```python
from build123d import *

# Parameters (mm, degrees)
BOSS_EXTRUDE1_DEPTH = 2.54
BOSS_EXTRUDE2_DEPTH = 6.35


with BuildPart() as part:
    # Sketch1 → Revolve1 (revolve)
    with BuildSketch(Plane.XY):
        with BuildLine():
            Line((0, -13.880770422), (0, -18.033881925))
            Line((0, -18.033881925), (17.78, -18.033881925))
            Line((17.78, -18.033881925), (17.78, -8.528719197))
            Line((17.78, -8.528719197), (15.24, -8.528719197))
            Line((15.24, -8.528719197), (15.24, -15.493881925))
            Line((15.24, -15.493881925), (12.7, -15.493881925))
            ThreePointArc((12.7, -15.493881925), (6.401018058, -14.285661851), (0, -13.880770422))
        make_face()
    revolve(axis=Axis((0, -13.880770422, 0), (0, -1, 0)))

    # Sketch2 → Boss-Extrude1 (add)
    with BuildSketch(Plane.XZ.offset(18.033881925)):
        Polygon((28.413494599, 0), (8.780252701, 27.022839189), (-22.987, 16.701033091), (-22.987, -16.701033091), (8.780252701, -27.022839189), align=None)
    extrude(amount=-BOSS_EXTRUDE1_DEPTH)

    # Sketch3 → Boss-Extrude2 (add)
    with BuildSketch(Plane(origin=(0, -15.493881925, 0), x_dir=(1, 0, 0), z_dir=(0, 1, 0))):
        Polygon((28.413494599, 0), (8.780252701, 27.022839189), (-22.987, 16.701033091), (-22.987, -16.701033091), (8.780252701, -27.022839189), align=None)
        Polygon((25.273881936, 0), (7.810059032, 24.036890107), (-20.447, 14.85561507), (-20.447, -14.85561507), (7.810059032, -24.036890107), align=None, mode=Mode.SUBTRACT)
    extrude(amount=BOSS_EXTRUDE2_DEPTH)


solid = part.part
```
Read the model definition and answer for the solid it produces. Units are mm, in the model's axes. A direction names the side the tool comes from. Round coordinates to 2 decimals unless told otherwise and drop trailing zeros. Write each loop counter-clockwise with the first axis right and the second up, starting at its lowest first coordinate (ties: lowest second). Pieces come first, ordered by that corner, then holes. Notation, with made-up numbers: (22, 59.5) - (39, 59.5) arc R19 ccw to (39, 71.5) - close; hole circle Ø8 at (75.5, -35.5). An arc over 180 degrees is marked (long way). One line per item, written item: value.
Q1. Each of these flat-tipped pins is pushed along its axis until it touches: P1, Ø13.5, axis at x = 3.5, z = 5, coming from the +Y side; P2, Ø1.5, axis at x = 1, y = -13, coming from the +Z side; P3, Ø5, axis at y = -13, z = -7.5, coming from the +X side. Where does it stop, or does it pass through?
The answers:
P1: stops at y = -13.88
P2: stops at z = 24.74
P3: stops at x = 24.78
Q2. Find section C-C (z = -2). Determine the outline of the cut face in (x, y), and give its area (3 significant figures).
The answers:
outline: (-22.99, -18.03) - (26.96, -18.03) - (26.96, -9.14) - (23.82, -9.14) - (23.82, -15.49) - (17.67, -15.49) - (17.67, -8.53) - (15.11, -8.53) - (15.11, -15.49) - (12.54, -15.49) arc R50.76 ccw to (-12.54, -15.49) - (-15.11, -15.49) - (-15.11, -8.53) - (-17.67, -8.53) - (-17.67, -15.49) - (-20.45, -15.49) - (-20.45, -9.14) - (-22.99, -9.14) - close
area: 225 mm2
Q3. Which of the six approach directions +Z, -Z, +X, -X, +Y, -Y give full straight-line access (tool end or side, diameter ignored) to faces 1 (the flat face through (-8, -8.529, 13.3)), 2 (the cylindrical face through (-3.3, -12.06, -14.88))?
The answers:
face 1: +Z, -Z, +X, -X, +Y
face 2: +Y
Q4. Find section A-A (y = -10.5). Determine the outline of the cut face in (x, z), and give its area (3 significant figures).
The answers:
outline: (-22.99, -16.7) - (8.78, -27.02) - (28.41, 0) - (8.78, 27.02) - (-22.99, 16.7) - close; circle Ø35.56 at (0, 0); hole (-20.45, -14.86) - (7.81, -24.04) - (25.27, 0) - (7.81, 24.04) - (-20.45, 14.86) - close; hole circle Ø30.48 at (0, 0)
area: 664 mm2
Q5. Find section D-D (x = 23.5). Determine the outline of the cut face in (y, z).
The answers:
outline: (-18.03, -6.76) - (-9.14, -6.76) - (-9.14, -2.44) - (-15.49, -2.44) - (-15.49, 2.44) - (-9.14, 2.44) - (-9.14, 6.76) - (-18.03, 6.76) - close
Q6. Straight lines are drawn through the part: line 1 (Z direction, x = -10, y = -9.75); line 2 (X direction, y = -10.5, z = -12); line 3 (X direction, y = -15, z = 12.5). For each, find the intervals that lie inside material, in ascending order. Write a range as from..to.
The answers:
line 1: z = -20.92..-18.25, -14.7..-11.5, 11.5..14.7, 18.25..20.92
line 2: x = -22.99..-20.45, -13.12..-9.39, 9.39..13.12, 16.56..19.69
line 3: x = -22.99..-20.45, -12.64..-8.72, 8.72..12.64, 16.19..19.33
Q7. Find section B-B (x = 14.5). Determine the outline of the cut face in (y, z).
The answers:
outline: (-18.03, -19.15) - (-9.14, -19.15) - (-9.14, -14.83) - (-15.49, -14.83) - (-15.49, -10.29) - (-8.53, -10.29) - (-8.53, -4.69) - (-15.49, -4.69) - (-15.49, 4.69) - (-8.53, 4.69) - (-8.53, 10.29) - (-15.49, 10.29) - (-15.49, 14.83) - (-9.14, 14.83) - (-9.14, 19.15) - (-18.03, 19.15) - close
Q8. For a pull along X with two mould halves and no side action, classify faces 3 (the flat face through (16.664, -12.363, -11.85)), 4 (the flat face through (18.734, -13.651, -13.322)), 5 (the flat face through (-7.3, -13.7, 21.8)) as pulls with the +X half, pulls with the -X half, needs draft (parallel to the pull), parting line crosses it, or undercut.
The answers:
face 3: undercut
face 4: pulls with the +X half
face 5: pulls with the -X half
